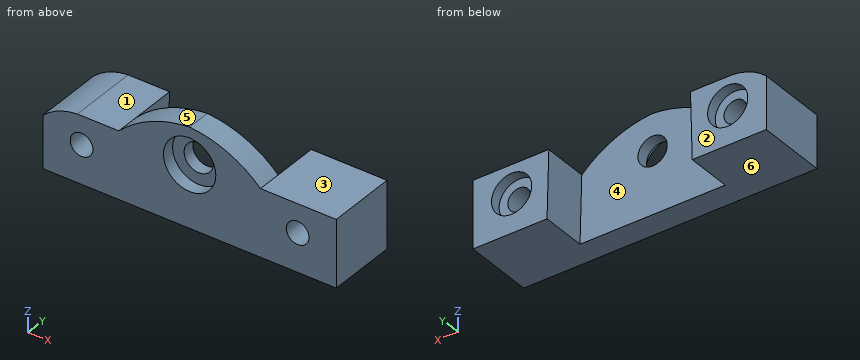
from build123d import *

# Parameters (mm, degrees)
SKETCH1_W           = 42
SKETCH1_H           = 10
SKETCH1_R           = 1.625
BOSS_EXTRUDE1_DEPTH = 10
SKETCH2_R           = 10.152178523
CUT_EXTRUDE2_DEPTH  = 6.5
CUT_EXTRUDE3_DEPTH  = 10
SKETCH4_R           = 2.875
CUT_EXTRUDE4_DEPTH  = 1.5
CUT_EXTRUDE5_DEPTH  = 8
BOSS_EXTRUDE6_DEPTH = 3.5
SKETCH10_R          = 2.1
CUT_EXTRUDE6_DEPTH  = 4.5
CUT_EXTRUDE8_DEPTH  = 10
SKETCH13_R          = 3.75
CUT_EXTRUDE9_DEPTH  = 1.8


with BuildPart() as part:
    # Sketch1 → Boss-Extrude1 (new body)
    with BuildSketch(Plane(origin=(0, 0, 0), x_dir=(1, 0, 0), z_dir=(0, 1, 0))):
        Rectangle(SKETCH1_W, SKETCH1_H)
        with Locations((-15.475, -0.525)):
            Circle(SKETCH1_R, mode=Mode.SUBTRACT)
        with Locations((15.475, -0.525)):
            Circle(SKETCH1_R, mode=Mode.SUBTRACT)
    extrude(amount=BOSS_EXTRUDE1_DEPTH)

    # Sketch2 → Cut-Extrude2 (cut)
    with BuildSketch(Plane(origin=(0, 10, 0), x_dir=(1, 0, 0), z_dir=(0, 1, 0))):
        with Locations((0, -5)):
            Circle(SKETCH2_R)
    extrude(amount=-CUT_EXTRUDE2_DEPTH, mode=Mode.SUBTRACT)

    # Sketch3 → Cut-Extrude3 (cut, symmetric)
    with BuildSketch(Plane(origin=(0, 3.5, 0), x_dir=(1, 0, 0), z_dir=(0, 1, 0))):
        Polygon((-21, -5), (21, -5), (21, -4.605153404), (9.605793631, -4.605153404), (9.605793631, -4.916952006), (-9.605793631, -4.916952006), (-9.605793631, -4.605153404), (-21, -4.605153404), (-21, -4.916952006), align=None)
    extrude(amount=CUT_EXTRUDE3_DEPTH, both=True, mode=Mode.SUBTRACT)

    # Sketch4 → Cut-Extrude4 (cut)
    with BuildSketch(Plane(origin=(0, 10, 0), x_dir=(1, 0, 0), z_dir=(0, 1, 0))):
        with Locations((-15.475, -0.525)):
            Circle(SKETCH4_R)
        with Locations((15.475, -0.525)):
            Circle(SKETCH4_R)
    extrude(amount=-CUT_EXTRUDE4_DEPTH, mode=Mode.SUBTRACT)

    # Sketch6 → Cut-Extrude5 (cut)
    with BuildSketch(Plane(origin=(0, 3.5, 0), x_dir=(1, 0, 0), z_dir=(0, 1, 0))):
        with BuildLine():
            Line((-10.144497274, -4.605153404), (-10.396714549, 5))
            Line((-10.396714549, 5), (-1.751207804, 5))
            ThreePointArc((-1.751207804, 5), (-7.644716659, 1.6801973), (-10.144497274, -4.605153404))
        make_face()
        with BuildLine():
            Line((10.144497274, -4.605153404), (10.396714549, 5))
            Line((10.396714549, 5), (1.751207804, 5))
            ThreePointArc((1.751207804, 5), (7.644716659, 1.6801973), (10.144497274, -4.605153404))
        make_face()
    extrude(amount=CUT_EXTRUDE5_DEPTH, mode=Mode.SUBTRACT)

    # Sketch9 → Boss-Extrude6 (add)
    with BuildSketch(Plane(origin=(0, 0, 0), x_dir=(1, 0, 0), z_dir=(0, 1, 0))):
        with BuildLine():
            Line((-10.144497274, -4.605153404), (-9.605793631, -4.605153404))
            Line((-9.605793631, -4.605153404), (-9.605793631, -4.916952006))
            Line((-9.605793631, -4.916952006), (9.605793631, -4.916952006))
            Line((9.605793631, -4.916952006), (9.605793631, -4.605153404))
            Line((9.605793631, -4.605153404), (10.144497274, -4.605153404))
            ThreePointArc((10.144497274, -4.605153404), (5.480668968, -7.794295111), (0, -9.166952006))
            ThreePointArc((0, -9.166952006), (-5.480668968, -7.794295111), (-10.144497274, -4.605153404))
        make_face()
    extrude(amount=BOSS_EXTRUDE6_DEPTH)

    # Sketch10 → Cut-Extrude6 (cut)
    with BuildSketch(Plane(origin=(0, 3.5, 0), x_dir=(1, 0, 0), z_dir=(0, 1, 0))):
        with Locations((0, -3.9)):
            Circle(SKETCH10_R)
    extrude(amount=-CUT_EXTRUDE6_DEPTH, mode=Mode.SUBTRACT)

    # Sketch12 → Cut-Extrude8 (cut)
    with BuildSketch(Plane(origin=(0, 10, 0), x_dir=(1, 0, 0), z_dir=(0, 1, 0))):
        with BuildLine():
            Line((-21, -4.605153404), (-21, -2.499927291))
            ThreePointArc((-21, -2.499927291), (-18.716787092, -3.977228829), (-16.070810572, -4.605153404))
            Line((-16.070810572, -4.605153404), (-21, -4.605153404))
        make_face()
    extrude(amount=-CUT_EXTRUDE8_DEPTH, mode=Mode.SUBTRACT)

    # Sketch13 → Cut-Extrude9 (cut)
    with BuildSketch(Plane.XZ):
        with Locations((0, 3.9)):
            Circle(SKETCH13_R)
    extrude(amount=-CUT_EXTRUDE9_DEPTH, mode=Mode.SUBTRACT)


solid = part.part
For this review, take the finished solid that the model builds, in its own axes (mm). Face numbers are marked on the shaded views. A direction names the side the tool comes from. Round coordinates to 2 decimals unless told otherwise and drop trailing zeros. Loops run counter-clockwise (first coordinate to the right, second up) from the corner with the lowest first, then second, coordinate; pieces in that order, holes last. Notation, with made-up numbers: (-19.75, 24) - (22.25, 24) arc R16 cw to (22.25, 41) - close; hole circle Ø8 at (-32.75, 56). An arc over 180 degrees is marked (long way). Use one line per item in the form item = value.
Item 1: Consider section B-B on z = 3.9. Write out the cut boundary in (x, y).
Answers:
outline = (-18.89, 0) - (-3.75, 0) - (-3.75, 1.8) - (-2.1, 1.8) - (-2.1, 3.5) - (-10.16, 3.5) - (-10.16, 10) - (-18.89, 10) - close; (2.1, 1.8) - (3.75, 1.8) - (3.75, 0) - (21, 0) - (21, 10) - (10.16, 10) - (10.16, 3.5) - (2.1, 3.5) - close
Item 2: Consider section A-A on y = 4. State how many separate pieces and enclosed holes the cut face has, then the cut area to 3 significant figures.
Answers:
separate_pieces = 2
enclosed_holes = 2
area = 186 mm^2
Item 3: Clearance check with flat-ended pins moving along their axes: P1, Ø7, axis at x = 0, z = 3.9, coming from the -Y side; P2, Ø4.5, axis at x = -15.475, z = 0.525, coming from the -Y side; P3, Ø1.8, axis at x = -14, y = 5.5, coming from the +Z side; P4, Ø1.7, axis at x = 14.5, z = 0, coming from the +Y side. State where each tip first meets the part, or that it passes through.
Answers:
P1 = 1.8
P2 = 0
P3 = 4.61
P4 = 8.5
Item 4: Consider section C-C on x = -4.5. Write out the cut boundary in (y, z).
Answers:
outline = (0, -5) - (3.5, -5) - (3.5, 8.2) - (0, 8.2) - close
Item 5: Tool access review of the marked faces 1, 2 and 3: name each direction out of +Z, -Z, +X, -X, +Y, -Y from which nothing blocks a thin tool from reaching the whole face with its end or side.
Answers:
face_1 = +Z, -X, +Y, -Y
face_2 = +Z, -Z, +X, -X, +Y
face_3 = +Z, +X, +Y, -Y
Item 6: Mouldability with a two-part tool opening along X and no side actions: class the marked faces 4, 5 and 6 as +X half, -X half, draft (parallel to the pull), parting line (faces both ways), or undercut.
Answers:
face_4 = undercut
face_5 = -X half
face_6 = draft
Item 7: For line 1 (X direction, y = 9.25, z = 0.5); line 2 (X direction, y = 2, z = 1); line 3 (X direction, y = 5.25, z = 2), list the stretches that pass through material, from the lowest coordinate up.
Answers:
line_1 = -21 to -18.35, -12.6 to -10.25, 10.25 to 12.6, 18.35 to 21
line_2 = -21 to -17.03, -13.92 to 13.92, 17.03 to 21
line_3 = -21 to -16.16, -14.79 to -10.21, 10.21 to 14.79, 16.16 to 21
